```python
from build123d import *

# Parameters (mm, degrees)
F1_DEPTH = 35
F2_DEPTH = 12.5
F3_W     = 55
F3_H     = 55
F4_DEPTH = 22.5
F5_R     = 22.5
F6_DEPTH = 60
F7_R     = 5
F8_R     = 1


with BuildPart() as f1:
    # F0 (on Top) → F1 (new body, symmetric)
    with BuildSketch(Plane.XY):
        Polygon((-10.1801488287, 27.5), (-27.5, 27.5), (-27.5, 10.1801488287), (-27.5, -10.1801488287), (-27.5, -27.5), (-14.1, -27.5), (14.1, -27.5), (27.5, -27.5), (27.5, -10.1801488287), (27.5, 10.1801488287), (27.5, 27.5), (10.1801488287, 27.5), align=None)
    extrude(amount=F1_DEPTH, both=True)

    # F0 (on Top) → F2 (join, symmetric)
    with BuildSketch(Plane.XY):
        Polygon((-12, 32.5), (-10.1801488287, 27.5), (10.1801488287, 27.5), (12, 32.5), align=None)
        Polygon((-27.5, -10.1801488287), (-27.5, 10.1801488287), (-32.5, 12), (-32.5, -12), align=None)
        Polygon((-14.1, -27.5), (-27.5, -27.5), (-27.5, -37.6), (-10.4239006339, -37.6), align=None)
        Polygon((27.5, -27.5), (14.1, -27.5), (10.4239006339, -37.6), (27.5, -37.6), align=None)
        Polygon((32.5, 12), (27.5, 10.1801488287), (27.5, -10.1801488287), (32.5, -12), align=None)
    extrude(amount=F2_DEPTH, both=True)

    # F3 (on face) → F4 (join, through all)
    with BuildSketch(Plane(origin=(0, 0, -35), x_dir=(1, 0, 0), z_dir=(0, 0, -1))):
        Rectangle(F3_W, F3_H)
        Polygon((27.5, 27.5), (27.5, -27.5), (-27.5, -27.5), (-27.5, 27.5), (-32.5, 27.5), (-32.5, -32.5), (32.5, -32.5), (32.5, 27.5), align=None)
    extrude(amount=-F4_DEPTH)

    # F5 (on face) → F6 (cut)
    with BuildSketch(Plane.XY.offset(35)):
        Circle(F5_R)
    extrude(amount=-F6_DEPTH, mode=Mode.SUBTRACT)

    # F7
    f7_edges = [f1.edges().sort_by_distance(p)[0] for p in [
        (-27.5, -27.5, 23.75),
        (-32.5, -27.5, -23.75),
        (27.5, -27.5, 23.75),
        (32.5, -27.5, -23.75),
        (27.5, 27.5, 11.25),
        (32.5, 32.5, -23.75),
        (-27.5, 27.5, 11.25),
        (-32.5, 32.5, -23.75),
        (0, -27.5, -35),
        (0, 32.5, -35),
        (32.5, 2.5, -35),
        (-32.5, 2.5, -35),
    ]]
    fillet(f7_edges, radius=F7_R)

    # F8
    f8_edges = [f1.edges().sort_by_distance(p)[0] for p in [
        (32.5, 12, 0),
        (32.5, -12, 0),
        (10.423901, -37.6, 0),
        (-10.423901, -37.6, 0),
        (-32.5, -12, 0),
        (-32.5, 12, 0),
        (-12, 32.5, 0),
        (12, 32.5, 0),
    ]]
    fillet(f8_edges, radius=F8_R)


solid = f1.part
```
Can you work these out from the model? Positions are in its coordinate system, mm. A direction names the side the tool comes from. Give positions to 0.01 mm unless a question says otherwise; leave off trailing zeros. Write each loop counter-clockwise with the first axis right and the second up, starting at its lowest first coordinate (ties: lowest second). Pieces come first, ordered by that corner, then holes. Notation, with made-up numbers: (-1, 39) -> (45, 39) arc R33 cw to (45, 73) -> close; hole circle Ø4 at (-7, -16). An arc over 180 degrees is marked (long way). Write item = value, one per line.
(1) Suppose I cut it at B-B on x = 0. Write out the boundary of the cut face in (y, z).
Worked out:
outline = (-27.5, -30) arc R5 ccw to (-22.5, -35) -> (27.5, -35) arc R5 ccw to (32.5, -30) -> (32.5, 12.5) -> (27.5, 12.5) -> (27.5, 35) -> (22.5, 35) -> (22.5, -25) -> (-22.5, -25) -> (-22.5, 35) -> (-27.5, 35) -> close
(2) Suppose I cut it at C-C on y = 0. Write out the boundary of the cut face in (x, z).
Worked out:
outline = (-32.5, -30) arc R5 ccw to (-27.5, -35) -> (27.5, -35) arc R5 ccw to (32.5, -30) -> (32.5, 12.5) -> (27.5, 12.5) -> (27.5, 35) -> (22.5, 35) -> (22.5, -25) -> (-22.5, -25) -> (-22.5, 35) -> (-27.5, 35) -> (-27.5, 12.5) -> (-32.5, 12.5) -> close
(3) Thinking about a two-plate mould opening in Y: for faces 5 (the face through (-27.5, -7, 17)), 6 (the face through (-12.5, -31.9, -0.2)), 7 (the face through (-31.07, -26, -21.13)), which applies, released by +Y, released by -Y, zero draft, split by the parting line, or undercut?
Worked out:
face_5 = zero draft
face_6 = undercut
face_7 = released by -Y
(4) I'm going to push flat-ended pins straight in: P1, Ø1, axis at y = -0.5, z = 21.5, coming from the +X side; P2, Ø10, axis at x = 12, z = 3, coming from the +Y side; P3, Ø12, axis at y = -28, z = -3, coming from the -X side; P4, Ø5, axis at x = 21.5, y = -31, coming from the -Z side. Where does each tip first touch, or does it pass through?
Worked out:
P1 = 27.5
P2 = 32.5
P3 = -27.5
P4 = -12.5
(5) For faces 1 (the face through (-19, -32, -12.5)), 2 (the face through (-29.355, -10.855, -0.175)), 3 (the face through (10.837, 29.303, -0.175)), 4 (the face through (-26, -26.07, 23.91)), which set-ups out of +Z, -Z, +X, -X, +Y, -Y let a thin tool reach every point of the face, with its end or its side?
Worked out:
face_1 = -Z, +X, -X, -Y
face_2 = +Z, -Y
face_3 = +Z, +X
face_4 = +Z, -X, -Y
(6) Suppose I cut it at D-D on y = 9. Write out the boundary of the cut face in (x, z), then the cut area to 3 significant figures.
Worked out:
outline = (-32.5, -30) arc R5 ccw to (-27.5, -35) -> (27.5, -35) arc R5 ccw to (32.5, -30) -> (32.5, 12.5) -> (27.5, 12.5) -> (27.5, 35) -> (20.62, 35) -> (20.62, -25) -> (-20.62, -25) -> (-20.62, 35) -> (-27.5, 35) -> (-27.5, 12.5) -> (-32.5, 12.5) -> close
area = 1,840 mm^2
(7) I need wall thicknesses on probe 1 along Y at (x, z) = (0, -1); probe 2 along Y at (x, z) = (15, 17.5); probe 3 along Z at (x, y) = (-6, -9). Which ranges of each line are inside material? Lowest first, please. Write a range as from..to.
Worked out:
probe_1 = -27.5..-22.5, 22.5..32.5
probe_2 = -27.5..-16.77, 16.77..27.5
probe_3 = -35..-25
